The drawing under review shows one solid part. Ordinate dimensions are in mm from its lowest x, y, z. A direction names the side the tool comes from. Coordinates: 2 decimals unless noted, no trailing zeros. Order: outer loops, then holes, each group sorted by start corner. A loop starts at its lowest first (then second) coordinate and runs counter-clockwise, first axis right, second up.
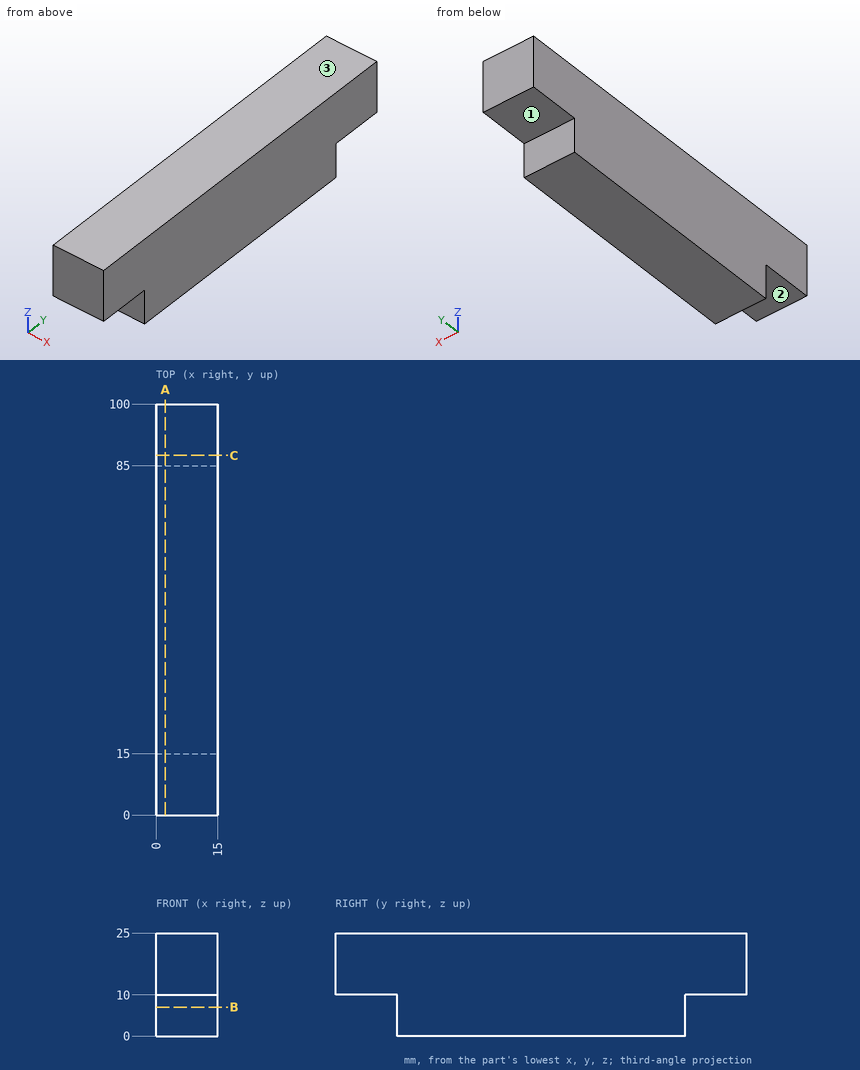
1. Machinability: for the marked faces 1, 2 and 3, which of the approach directions +Z, -Z, +X, -X, +Y, -Y give a long, thin tool a straight path to every point of the face, cutting with its end or side? Answer none if there is none.
Answer below:
face 1: -Z, +X, -X, +Y
face 2: -Z, +X, -X, -Y
face 3: +Z, +X, -X, +Y, -Y
2. Take a section at B-B, the plane z = 7. Give the boundary of the cut face in (x, y), plus the area to 3 significant figures.
Answer below:
outline: (0, 15) - (15, 15) - (15, 85) - (0, 85) - close
area: 1,050 mm2
3. Take a section at A-A, the plane x = 2.25. Give the boundary of the cut face in (y, z), plus the area to 3 significant figures.
Answer below:
outline: (0, 10) - (15, 10) - (15, 0) - (85, 0) - (85, 10) - (100, 10) - (100, 25) - (0, 25) - close
area: 2,200 mm2
4. Take a section at C-C, the plane y = 87.5. Give the boundary of the cut face in (x, z), plus the area to 3 significant figures.
Answer below:
outline: (0, 10) - (15, 10) - (15, 25) - (0, 25) - close
area: 225 mm2
5. To check wall thickness, follow L1, parallel to Y at x = 3, z = 4.75; L2, parallel to Z at x = 11, y = 12. State the ranges of each line that lie inside material, in increasing order.
Answer below:
L1: y = 15 to 85
L2: z = 10 to 25
6. Clearance check with a flat-ended pin moving along its axis: pin 1 Ø2 at (x, y) = (2, 89.5) entering from -Z. State where the tip first meets the part, or that it passes through.
Answer below:
pin 1: stops at z = 10
